from build123d import *

# Parameters (mm, degrees)
SKETCH_1_R      = 4
SKETCH_1_R_2    = 1.5
EXTRUDE_1_DEPTH = 2
SKETCH_2_R      = 4.6
SKETCH_2_R_2    = 4
EXTRUDE_2_DEPTH = 0.9
CHAMFER_1_SIZE  = 0.1


with BuildPart() as part:
    # 草图1 → 凸台-拉伸1 (new body, symmetric)
    with BuildSketch(Plane.XY):
        Circle(SKETCH_1_R)
        Circle(SKETCH_1_R_2, mode=Mode.SUBTRACT)
    extrude(amount=EXTRUDE_1_DEPTH, both=True)

    # 草图2 → 凸台-拉伸2 (add)
    with BuildSketch(Plane(origin=(0, 0, -2), x_dir=(-1, 0, 0), z_dir=(0, 0, -1))):
        Circle(SKETCH_2_R)
        Circle(SKETCH_2_R_2, mode=Mode.SUBTRACT)
    extrude(amount=-EXTRUDE_2_DEPTH)

    # 倒角1
    chamfer_1_edges = [part.edges().sort_by_distance(p)[0] for p in [
        (4.6, 0, -1.1),
        (4.6, 0, -2),
        (-4, 0, 2),
        (-1.5, 0, -2),
        (-1.5, 0, 2),
    ]]
    chamfer(chamfer_1_edges, length=CHAMFER_1_SIZE)


solid = part.part
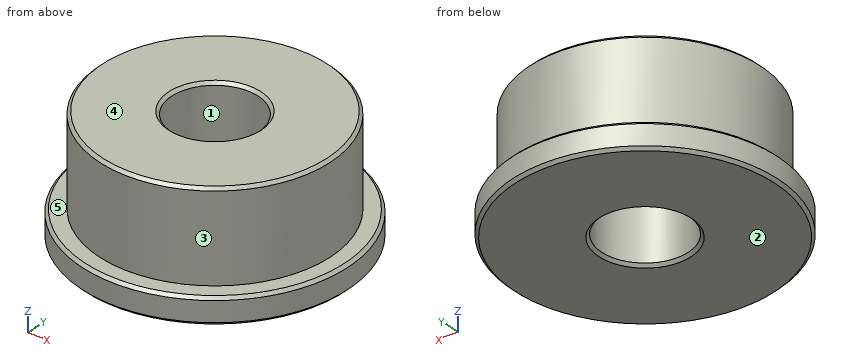
Could you check a few things on this model? Use its own coordinates, in mm. Face numbers are marked on the shaded views. A direction names the side the tool comes from. Coordinates: 2 decimals unless noted, no trailing zeros. Write each loop counter-clockwise with the first axis right and the second up, starting at its lowest first coordinate (ties: lowest second). Pieces come first, ordered by that corner, then holes. Notation, with made-up numbers: (60, 36) - (97, 36) arc R11 cw to (97, 56) - close; hole circle Ø3 at (23.5, 51.25). An arc over 180 degrees is marked (long way). Write item = value, one per line.
1) Please list where these lines run through material, in increasing order: line 1 (Y direction, x = 0, z = 0); line 2 (Z direction, x = -3.5, y = -2.75); line 3 (Y direction, x = 0.5, z = 0.6). Write a range as [from, to].
Result set:
line_1 = [-4, -1.5], [1.5, 4]
line_2 = [-2, -1.1]
line_3 = [-3.97, -1.41], [1.41, 3.97]
2) We'd pull the mould along Y, two halves only. Please class the marked faces 1, 2 and 3: +Y half, -Y half, draft (parallel to the pull), parting line (faces both ways), or undercut.
Result set:
face_1 = undercut
face_2 = draft
face_3 = parting line
3) Will this pin go through, and if not, where does the flat tip stop? pin 1 Ø1.5 at (x, z) = (-3, -1) entering from -Y.
Result set:
pin_1 = -4
4) Suppose I cut it at B-B on z = 0.8. Please give me the cut outline in (x, y).
Result set:
outline = circle Ø8 at (0, 0); hole circle Ø3 at (0, 0)
5) Suppose I cut it at A-A on x = 0. Please give me the cut outline in (y, z), plus the area to 3 significant figures.
Result set:
outline = (-4.6, -1.9) - (-4.5, -2) - (-1.6, -2) - (-1.5, -1.9) - (-1.5, 1.9) - (-1.6, 2) - (-3.9, 2) - (-4, 1.9) - (-4, -1.1) - (-4.5, -1.1) - (-4.6, -1.2) - close; (1.5, -1.9) - (1.6, -2) - (4.5, -2) - (4.6, -1.9) - (4.6, -1.2) - (4.5, -1.1) - (4, -1.1) - (4, 1.9) - (3.9, 2) - (1.6, 2) - (1.5, 1.9) - close
area = 21.0 mm2
6) For the marked faces 4 and 5, which set-ups out of +Z, -Z, +X, -X, +Y, -Y let a thin tool reach every point of the face, with its end or its side?
Result set:
face_4 = +Z, +X, -X, +Y, -Y
face_5 = +Z
